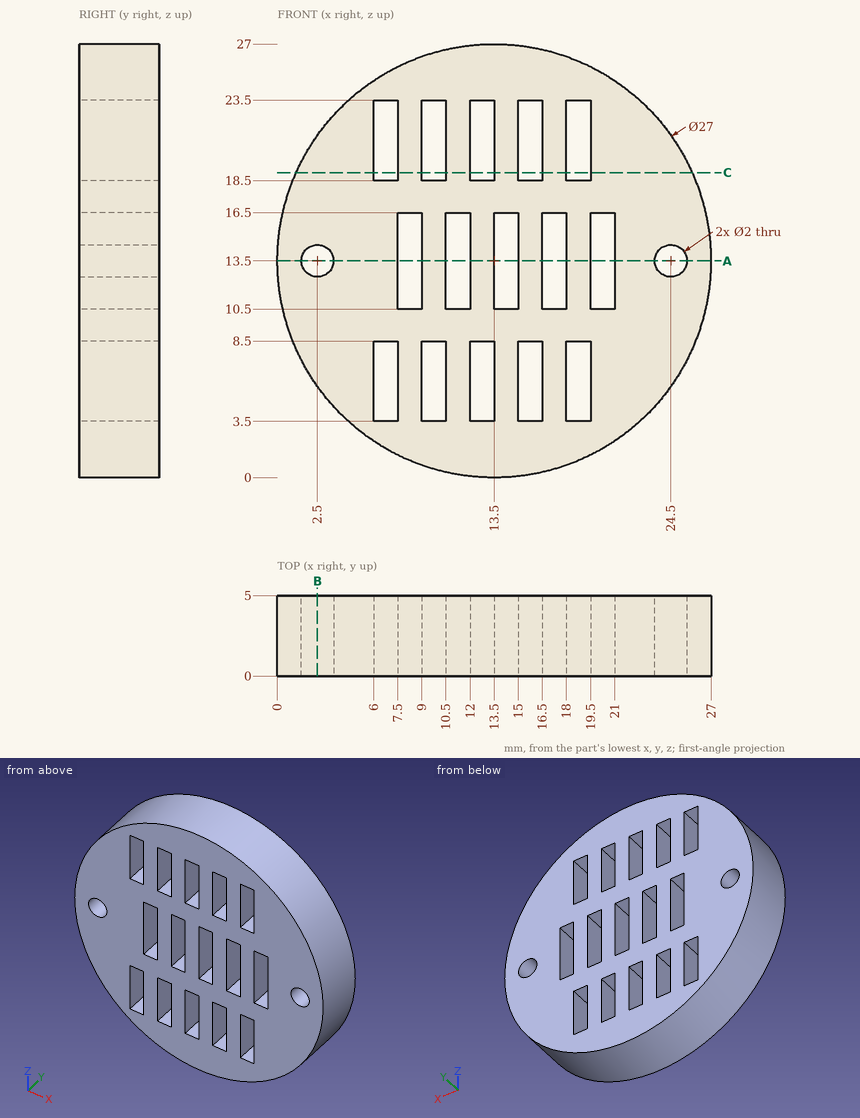
Verification items for this drawing (mm, ordinates from the low corner). Coordinates: 2 decimals unless noted, no trailing zeros. Write each loop counter-clockwise with the first axis right and the second up, starting at its lowest first coordinate (ties: lowest second). Pieces come first, ordered by that corner, then holes. Notation, with made-up numbers: M 65,-27.5 L 115,-27.5 A25 ccw 115,-6.5 Z; hole C 42.5,-29 d4. An arc over 180 degrees is marked long. One line per item, written item: value. Start each with the question number.
(1) Sectioned sample at A-A, the plane z = 13.5. State how many separate pieces and enclosed holes the cut face has, and give its area (3 significant figures).
(2) Sectioned sample at B-B, the plane x = 2.5. Enter the section's corners in (y, z).
(3) Depth check by flat-ended pin: pin 1 (2.5 mm diameter, centred on y = 1.5, z = 5, fed in from +X); pin 2 (1.2 mm diameter, centred on x = 17, y = 2.5, fed in from +Z); pin 3 (1.6 mm diameter, centred on x = 9.5, y = 3, fed in from +Z). Enter the tip coordinate at first touch or a pass-through.
(4) Sectioned sample at C-C, the plane z = 19. Enter the section's corners in (x, y), and give its area (3 significant figures).
(5) Scan lines: line 1 along X through (y, z) = (3.8, 7.25); line 2 along X through (y, z) = (1.25, 7); line 3 along Z through (x, y) = (19, 3.15). Record each from-to range of solid material in increasing order. Write a range as [from, to].
Filled sheet:
1. separate pieces: 8
1. enclosed holes: 0
1. area: 77.5 mm²
2. outline: M 0,5.67 L 5,5.67 L 5,12.5 L 0,12.5 Z; M 0,14.5 L 5,14.5 L 5,21.33 L 0,21.33 Z
3. pin 1: x = 24.89
3. pin 2: z = 26.68
3. pin 3: z = 26.62
4. outline: M 1.17,0 L 6,0 L 6,5 L 1.17,5 Z; M 7.5,0 L 9,0 L 9,5 L 7.5,5 Z; M 10.5,0 L 12,0 L 12,5 L 10.5,5 Z; M 13.5,0 L 15,0 L 15,5 L 13.5,5 Z; M 16.5,0 L 18,0 L 18,5 L 16.5,5 Z; M 19.5,0 L 25.83,0 L 25.83,5 L 19.5,5 Z
4. area: 85.8 mm²
5. line 1: [1.53, 6], [7.5, 9], [10.5, 12], [13.5, 15], [16.5, 18], [19.5, 25.47]
5. line 2: [1.67, 6], [7.5, 9], [10.5, 12], [13.5, 15], [16.5, 18], [19.5, 25.33]
5. line 3: [1.17, 3.5], [8.5, 18.5], [23.5, 25.83]
